Input: part model. Units: mm. Frame: model coordinates. A direction names the side the tool comes from. Give positions to 0.01 mm unless a question says otherwise; leave off trailing zeros. Loops run counter-clockwise (first coordinate to the right, second up) from the corner with the lowest first, then second, coordinate; pieces in that order, holes last. Notation, with made-up numbers: (-9, 82) -> (5, 82) arc R24 cw to (5, 118) -> close; hole circle Ø8 at (11, 44.5). An arc over 180 degrees is marked (long way). Use CSV: the item, a comma, the result in double quotes.
Autodesk Inventor part; units mm, degrees
ref_plane "YZ Plane" through (0, 0, 0) normal (1, 0, 0) x (0, 1, 0)
ref_plane "XZ Plane" through (0, 0, 0) normal (0, 1, 0) x (-1, 0, 0)
ref_plane "XY Plane" through (0, 0, 0) normal (0, 0, 1) x (1, 0, 0)
sketch "Esquisse1" plane through (0, 0, 0) normal (0, 0, 1) x (1, 0, 0)
  line L0 (-25, 25) -> (25, 25)
  line L1 (25, 25) -> (25, -25)
  line L2 (25, -25) -> (-25, -25)
  line L3 (-25, -25) -> (-25, 25)
  point P0 (0, 0)
  dimension "d0" = 50
  dimension "d1" = 25
  dimension "d2" = 50
  dimension "d3" = 25
extrude "Extrusion1" add sketch "Esquisse1" along normal blind 31
chamfer "Chanfrein1" distance 8 angle 45 4 edges at (25, 25, 15.5) (-25, 25, 15.5) (-25, -25, 15.5) (25, -25, 15.5)
sketch "Esquisse4" plane through (0, 0, 31) normal (0, 0, 1) x (1, 0, 0)
  line L0 (17, 25) -> (-17, 25)
  line L1 (-12, 25) -> (12, 25)
  line L2 (25, 17) -> (25, -17)
  line L3 (25, 12) -> (25, -12)
  line L4 (-17, -25) -> (17, -25)
  line L5 (12, -25) -> (-12, -25)
  line L6 (-25, 17) -> (-25, -17)
  line L7 (-25, -12) -> (-25, 12)
  line L8 (-25, 12) -> (-12, 25)
  line L9 (12, 25) -> (25, 12)
  line L10 (17, 25) -> (25, 17)
  line L11 (25, -12) -> (12, -25)
  line L12 (-12, -25) -> (-25, -12)
  point P0 (0, 0)
  dimension "d11" = 24
  dimension "d12" = 24
  dimension "d13" = 24
  dimension "d14" = 24
  dimension "d15" = 12
  dimension "d16" = 12
extrude "Extrusion3" add sketch "Esquisse4" along normal blind 31 contours L9 L2 L11 L4 L12 L6 L8 L0
sketch "Esquisse5" plane through (0, 0, 62) normal (0, 0, 1) x (1, 0, 0)
  line L0 (-27.5, 27.5) -> (27.5, 27.5)
  line L1 (27.5, 27.5) -> (27.5, -27.5)
  line L2 (27.5, -27.5) -> (-27.5, -27.5)
  line L3 (-27.5, -27.5) -> (-27.5, 27.5)
  point P0 (0, 0)
  dimension "d19" = 55
  dimension "d20" = 55
  dimension "d21" = 27.5
  dimension "d22" = 27.5
extrude "Extrusion4" add sketch "Esquisse5" along normal blind 6
sketch "Esquisse6" plane through (0, 0, 68) normal (0, 0, 1) x (1, 0, 0)
  circle A0 centre (0, 0) radius 20
  circle A1 centre (0, 0) radius 12.5
  dimension "d25" = 40
  dimension "d26" = 25
extrude "Extrusion5" add sketch "Esquisse6" along normal blind 2.5
sketch "Esquisse7" plane through (0, 0, 68) normal (0, 0, 1) x (1, 0, 0)
  circle A0 centre (0, 0) radius 4.5
  dimension "d29" = 9
extrude "Extrusion6" add sketch "Esquisse7" along normal blind 20
sketch "Esquisse8" plane through (0, 0, 68) normal (0, 0, 1) x (1, 0, 0)
  circle A0 centre (-22.2739, 22.2739) radius 2.9
  line L0 (-22.2739, 22.2739) -> (-27.5, 22.2739)
  line L1 (-27.5, 27.5) -> (-27.5, -27.5)
  line L2 (-22.2739, 22.2739) -> (-22.2739, 27.5)
  line L3 (27.5, 27.5) -> (-27.5, 27.5)
  circle A1 centre (-22.2739, -22.2739) radius 2.9
  circle A2 centre (22.2739, -22.2739) radius 2.9
  circle A3 centre (22.2739, 22.2739) radius 2.9
  point P0 (0, 0)
  dimension "d32" = 5.8
  dimension "d33" = 31.5
  dimension "d36" = 360
extrude "Extrusion7" cut sketch "Esquisse8" against normal blind 6 contours A0 L0 L2 | L2 L0 A0 | A1 | A2 | A3
chamfer "Chanfrein2" distance 3 angle 45 4 edges at (-27.5, 27.5, 65) (27.5, 27.5, 65) (27.5, -27.5, 65) (-27.5, -27.5, 65)
fillet "Congé1" radius 3 4 edges at (18.5, 18.5, 31) (18.5, -18.5, 31) (-18.5, 18.5, 31) (-18.5, -18.5, 31)
chamfer "Chanfrein3" distance 0.5 angle 45 1 edges at (-4.5, 0, 88)
equation "\"d2\" = d0"
equation "\"d12\" = d11"
equation "\"d13\" = d11"
equation "\"d14\" = d11"
equation "\"d20\" = d19"
properties part number "N2-0028-30-24" material "Aluminium 6061"
1) Section query D-D (z = 22). Return loops of the section in (x, y).
From the geometry:
outline,"(-25, -17) -> (-17, -25) -> (17, -25) -> (25, -17) -> (25, 17) -> (17, 25) -> (-17, 25) -> (-25, 17) -> close"
2) Section query A-A (y = 0). Return loops of the section in (x, z).
From the geometry:
outline,"(-27.5, 62) -> (-25, 62) -> (-25, 0) -> (25, 0) -> (25, 62) -> (27.5, 62) -> (27.5, 68) -> (20, 68) -> (20, 70.5) -> (12.5, 70.5) -> (12.5, 68) -> (4.5, 68) -> (4.5, 87.5) -> (4, 88) -> (-4, 88) -> (-4.5, 87.5) -> (-4.5, 68) -> (-12.5, 68) -> (-12.5, 70.5) -> (-20, 70.5) -> (-20, 68) -> (-27.5, 68) -> close"
3) Ray query, line 1 (X direction, y = -23, z = 64); line 2 (X direction, y = -15.5, z = 30.5); line 3 (Z direction, x = 16, y = -6.5). Return the intervals inside material, ascending.
From the geometry:
line 1,"x = -27.5 to -25.08, -19.47 to 19.47, 25.08 to 27.5"
line 2,"x = -25 to 25"
line 3,"z = 0 to 70.5"
4) Section query C-C (z = 66). Return loops of the section in (x, y).
From the geometry:
outline,"(-27.5, -24.5) -> (-24.5, -27.5) -> (24.5, -27.5) -> (27.5, -24.5) -> (27.5, 24.5) -> (24.5, 27.5) -> (-24.5, 27.5) -> (-27.5, 24.5) -> close; hole circle Ø5.8 at (-22.27, -22.27); hole circle Ø5.8 at (-22.27, 22.27); hole circle Ø5.8 at (22.27, -22.27); hole circle Ø5.8 at (22.27, 22.27)"
5) Mould query, pull axis Y, two halves, no side actions, for faces 6 (the flat face through (-21, 21, 16)), 7 (the cylindrical face through (11.923, -3.755, 69.232)), 8 (the flat face through (27.5, 0, 65)), 9 (the cylindrical face through (-19.2, -19.01, 31.9)). Classes: pulls with the +Y half, pulls with the -Y half, needs draft (parallel to the pull), parting line crosses it, or undercut.
From the geometry:
face 6,"pulls with the +Y half"
face 7,"undercut"
face 8,"needs draft"
face 9,"pulls with the -Y half"
6) Contact query for flat-ended pins moving along their axis: pin 1 (4 mm diameter, centred on x = -17, y = -3.5, fed in from +Z); pin 2 (12 mm diameter, centred on x = 13.5, z = 52, fed in from +Y); pin 3 (12 mm diameter, centred on x = -16.5, z = 38, fed in from -Y). Output: stop coordinate, or through.
From the geometry:
pin 1,"stops at z = 70.5"
pin 2,"stops at y = 25"
pin 3,"stops at y = -25"
7) Reachability of faces 1 (the flat face through (19, -18, 48)), 2 (the flat face through (21, -21, 15)), 3 (the cylindrical face through (23.61, 19.7, 65.04)), 4 (the flat face through (-25, 0, 31)), 5 (the flat face through (18, 19, 48)) from +Z, -Z, +X, -X, +Y, -Y: full face, straight path, thin tool, end or side. Return the list, or none.
From the geometry:
face 1,"+X, -Y"
face 2,"-Z, +X, -Y"
face 3,"+Z"
face 4,"-Z, -X, +Y, -Y"
face 5,"+X, +Y"
